```python
from build123d import *

# Parameters (mm, degrees)
EXTRUDE_1_DEPTH        = 22.5
SKETCH_3_W             = 17
SKETCH_3_H             = 0.2
CUT_EXTRUDE_1_DEPTH    = 0.5
HOLE_WIZARD_M2_1_D     = 1.6
HOLE_WIZARD_M2_1_DEPTH = 4.2
HOLE_WIZARD_M2_1_TIP   = 0.480688495


with BuildPart() as part:
    # 草图2 → 凸台-拉伸1 (new body)
    with BuildSketch(Plane.XY):
        Polygon((-8.5, 0), (8.5, 0), (8.5, -6.5), (3.5, -6.5), (3.5, -5.6), (2.7, -4.8), (3.5, -4), (3.5, -3.2), (-3.5, -3.2), (-3.5, -4), (-2.7, -4.8), (-3.5, -5.6), (-3.5, -6.5), (-8.5, -6.5), align=None)
    extrude(amount=EXTRUDE_1_DEPTH)

    # 草图3 → 切除-拉伸1 (cut)
    with BuildSketch(Plane(origin=(0, 0, 0), x_dir=(1, 0, 0), z_dir=(0, 1, 0))):
        with Locations((0, -17.65)):
            Rectangle(SKETCH_3_W, SKETCH_3_H)
        with Locations((0, -4.85)):
            Rectangle(SKETCH_3_W, SKETCH_3_H)
    extrude(amount=-CUT_EXTRUDE_1_DEPTH, mode=Mode.SUBTRACT)

    # M2 螺纹孔1
    with Locations(Plane(origin=(0, 0, 0), x_dir=(1, 0, 0), z_dir=(0, 1, 0))):
        with Locations((-6, -7.25), (6, -7.25), (6, -15.25), (-6, -15.25)):
            Hole(HOLE_WIZARD_M2_1_D / 2, depth=HOLE_WIZARD_M2_1_DEPTH)
            with Locations((0, 0, -(HOLE_WIZARD_M2_1_DEPTH + HOLE_WIZARD_M2_1_TIP / 2))):  # 118° drill point
                Cone(0, HOLE_WIZARD_M2_1_D / 2, HOLE_WIZARD_M2_1_TIP, mode=Mode.SUBTRACT)


solid = part.part
```
Source: CAD feature listing. Evaluate the final solid. Frame: model axes, mm. A direction names the side the tool comes from. Round coordinates to 2 decimals unless told otherwise and drop trailing zeros. Write each loop counter-clockwise with the first axis right and the second up, starting at its lowest first coordinate (ties: lowest second). Pieces come first, ordered by that corner, then holes. Notation, with made-up numbers: M -1.5,-36 L 28.5,-36 A24 cw 28.5,-11 Z; hole C 76,34 d3. An arc over 180 degrees is marked long. Use CSV: the item, a comma, the result in double quotes. Start each with the question number.
Q1. Pull-direction query (Z, two-part tool) for faces 5 (the face through (-6.03, -4.597, 15.386)), 6 (the face through (8.5, -3, 11)), 7 (the face through (0, -2, 0)), 8 (the face through (0, -2, 22.5)); classes: +Z half, -Z half, draft (parallel to the pull), parting line (faces both ways), or undercut.
Q2. Cut plane C-C on y = -2.25. Output: boundary loops of the cut face in (x, z), plus the area to 3 significant figures.
Q3. Line query: line 1 (Z direction, x = -6, y = -2.85); line 2 (X direction, y = -1.1, z = 15.25); line 3 (X direction, y = -3.25, z = 20). Output: solid intervals per line, ascending. Write a range as from..to.
Q4. Cut plane A-A on y = -0.25. Output: boundary loops of the cut face in (x, z), plus the area to 3 significant figures.
Q5. First-contact query: P1, Ø1, axis at x = 6, z = 15.25, coming from the +Y side; P2, Ø4, axis at x = -0.5, z = 4.5, coming from the -Y side. Flat tips, straight axial feed; report the tip coordinate or a pass-through.
Q6. Cut plane B-B on x = 3. Output: boundary loops of the cut face in (y, z).
Q7. Cut plane D-D on z = 9.25. Output: boundary loops of the cut face in (x, y).
Q8. Access query for faces 1 (the face through (-5.2, -2.1, 7.2)), 2 (the face through (-3.5, -6, 11)), 3 (the face through (0, -3.2, 11)), 4 (the face through (0, 0, 20)). Directions: +Z, -Z, +X, -X, +Y, -Y. A direction counts if a zero-diameter tool reaches every point of the face in a straight line with its end or side. Return the directions, or none.
Results found:
1,face 5,"undercut"
1,face 6,"draft"
1,face 7,"-Z half"
1,face 8,"+Z half"
2,outline,"M -8.5,0 L 8.5,0 L 8.5,22.5 L -8.5,22.5 Z; hole C -6,7.25 d1.6; hole C -6,15.25 d1.6; hole C 6,7.25 d1.6; hole C 6,15.25 d1.6"
2,area,"374 mm^2"
3,line 1,"0..6.45, 8.05..14.45, 16.05..22.5"
3,line 2,"-8.5..-6.8, -5.2..5.2, 6.8..8.5"
3,line 3,"-8.5..-3.5, 3.5..8.5"
4,outline,"M -8.5,0 L 8.5,0 L 8.5,4.75 L -8.5,4.75 Z; M -8.5,4.95 L 8.5,4.95 L 8.5,17.55 L -8.5,17.55 Z; M -8.5,17.75 L 8.5,17.75 L 8.5,22.5 L -8.5,22.5 Z; hole C -6,7.25 d1.6; hole C -6,15.25 d1.6; hole C 6,7.25 d1.6; hole C 6,15.25 d1.6"
4,area,"368 mm^2"
5,P1,"y = -4.38"
5,P2,"y = -3.2"
6,outline,"M -5.1,0 L -4.5,0 L -4.5,22.5 L -5.1,22.5 Z; M -3.2,0 L 0,0 L 0,4.75 L -0.5,4.75 L -0.5,4.95 L 0,4.95 L 0,17.55 L -0.5,17.55 L -0.5,17.75 L 0,17.75 L 0,22.5 L -3.2,22.5 Z"
7,outline,"M -8.5,-6.5 L -3.5,-6.5 L -3.5,-5.6 L -2.7,-4.8 L -3.5,-4 L -3.5,-3.2 L 3.5,-3.2 L 3.5,-4 L 2.7,-4.8 L 3.5,-5.6 L 3.5,-6.5 L 8.5,-6.5 L 8.5,0 L -8.5,0 Z"
8,face 1,"+Y"
8,face 2,"+Z, -Z, -Y"
8,face 3,"+Z, -Z"
8,face 4,"+Z, -Z, +X, -X, +Y"
